Verification items for the finished model (mm, model axes). Face numbers are marked on the shaded views. A direction names the side the tool comes from. Coordinates: 2 decimals unless noted, no trailing zeros. Loops run counter-clockwise (first coordinate to the right, second up) from the corner with the lowest first, then second, coordinate; pieces in that order, holes last. Notation, with made-up numbers: (-5, -15.5) - (22, -15.5) arc R28 ccw to (22, 11.5) - close; hole circle Ø8 at (-40, 37). An arc over 180 degrees is marked (long way). One line per item, written item: value. Start each with the question number.
(1) Gauge pin test, flat ends, axial feed: P1, Ø10, axis at x = 4.5, y = -4, coming from the -Z side; P2, Ø6, axis at x = 1.5, y = 10, coming from the -Z side. Record the tip position at first contact, or that the pin passes through.
(2) Section check D-D (x = -1.25). Record the boundary of the cut face in (y, z).
(3) Section check B-B (y = 20.5). Record the boundary of the cut face in (x, z).
(4) Section check A-A (z = -1.5). Record the boundary of the cut face in (x, y), plus the area to 4 significant figures.
(5) Draft check along X on the marked faces 1, 2, 3 and 4. Enter one of: +X half, -X half, draft (parallel to the pull), parting line (faces both ways), or undercut.
(6) Set-up check for the marked faces 5 and 6: record each of +Z, -Z, +X, -X, +Y, -Y from which the full face is reachable in a straight line by a thin tool's end or side.
(7) Thickness scan on probe 1 along Y at (x, z) = (-10, 3.6); probe 2 along X at (y, z) = (18.5, -2.5); probe 3 along X at (y, z) = (10, 3.55). Record the ranges inside material, lowest first. Write a range as [from, to].
(8) Section check C-C (z = 2). Record the boundary of the cut face in (x, y), plus the area to 3 significant figures.
```python
from build123d import *

# Parameters (mm, degrees)
F1_DEPTH = 23.85
F3_D     = 3.4
F3_DEPTH = 3.5
F3_TIP   = 1.0214630523


with BuildPart() as f1:
    # F0 (on Front) → F1 (new body, symmetric)
    with BuildSketch(Plane.XZ):
        Polygon((6, -5), (13.5, -5), (13.5, 5), (-13.5, 5), (-13.5, -5), (-6, -5), (-6, 1.5), (6, 1.5), align=None)
    extrude(amount=F1_DEPTH, both=True)

    # F3
    with Locations(Plane.XY.offset(5)):
        with Locations((10, 10), (10, -10), (-10, -10), (-10, 10)):
            Hole(F3_D / 2, depth=F3_DEPTH)
            with Locations((0, 0, -(F3_DEPTH + F3_TIP / 2))):  # 118° drill point
                Cone(0, F3_D / 2, F3_TIP, mode=Mode.SUBTRACT)


solid = f1.part
```
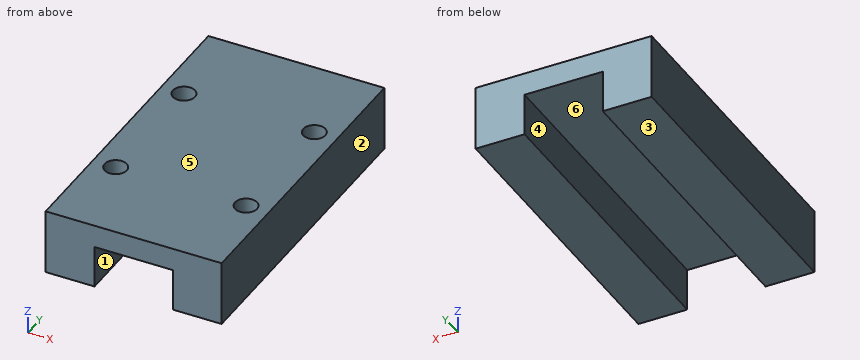
Responses:
1. P1: stops at z = -5
1. P2: stops at z = 1.5
2. outline: (-23.85, 1.5) - (23.85, 1.5) - (23.85, 5) - (-23.85, 5) - close
3. outline: (-13.5, -5) - (-6, -5) - (-6, 1.5) - (6, 1.5) - (6, -5) - (13.5, -5) - (13.5, 5) - (-13.5, 5) - close
4. outline: (-13.5, -23.85) - (-6, -23.85) - (-6, 23.85) - (-13.5, 23.85) - close; (6, -23.85) - (13.5, -23.85) - (13.5, 23.85) - (6, 23.85) - close
4. area: 715.5 mm²
5. face 1: undercut
5. face 2: +X half
5. face 3: draft
5. face 4: undercut
6. face 5: +Z, +X, -X, +Y, -Y
6. face 6: -Z, +Y, -Y
7. probe 1: y = [-23.85, -11.7], [-8.3, 8.3], [11.7, 23.85]
7. probe 2: x = [-13.5, -6], [6, 13.5]
7. probe 3: x = [-13.5, -11.7], [-8.3, 8.3], [11.7, 13.5]
8. outline: (-13.5, -23.85) - (13.5, -23.85) - (13.5, 23.85) - (-13.5, 23.85) - close; hole circle Ø3.4 at (-10, -10); hole circle Ø3.4 at (-10, 10); hole circle Ø3.4 at (10, -10); hole circle Ø3.4 at (10, 10)
8. area: 1,250 mm²
